Design review of the part shown in the three views and the two pictorial views. Dimensions are in mm from the part's minimum x, y and z. A direction names the side the tool comes from. Give positions to 0.01 mm unless a question says otherwise; leave off trailing zeros. Write each loop counter-clockwise with the first axis right and the second up, starting at its lowest first coordinate (ties: lowest second). Pieces come first, ordered by that corner, then holes. Notation, with made-up numbers: (-14, -37) -> (23, -37) arc R16 ccw to (23, -28) -> close; hole circle Ø10 at (67.25, 81.5). An arc over 180 degrees is marked (long way). Use CSV: the item, a comma, the result in double quotes.
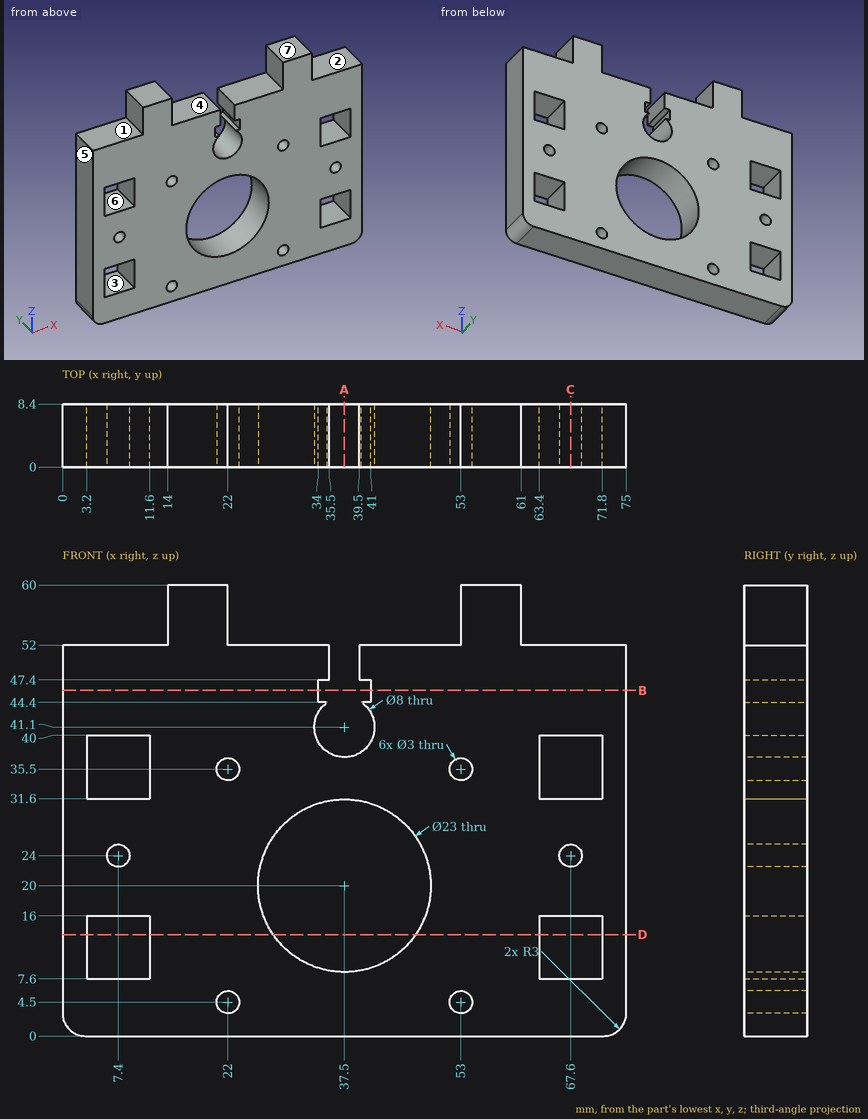
Q1. Consider section D-D (z = 13.5). Write out the cut boundary in (x, y).
Derived:
outline,"(0, 0) -> (3.2, 0) -> (3.2, 8.4) -> (0, 8.4) -> close; (11.6, 0) -> (28.01, 0) -> (28.01, 8.4) -> (11.6, 8.4) -> close; (46.99, 0) -> (63.4, 0) -> (63.4, 8.4) -> (46.99, 8.4) -> close; (71.8, 0) -> (75, 0) -> (75, 8.4) -> (71.8, 8.4) -> close"
Q2. Consider section C-C (x = 67.6). Write out the cut boundary in (y, z).
Derived:
outline,"(0, 0) -> (8.4, 0) -> (8.4, 7.6) -> (0, 7.6) -> close; (0, 16) -> (8.4, 16) -> (8.4, 22.5) -> (0, 22.5) -> close; (0, 25.5) -> (8.4, 25.5) -> (8.4, 31.6) -> (0, 31.6) -> close; (0, 40) -> (8.4, 40) -> (8.4, 52) -> (0, 52) -> close"
Q3. Consider section B-B (z = 46). Write out the cut boundary in (x, y).
Derived:
outline,"(0, 0) -> (34, 0) -> (34, 8.4) -> (0, 8.4) -> close; (41, 0) -> (75, 0) -> (75, 8.4) -> (41, 8.4) -> close"
Q4. Machinability: for the marked faces 1, 2 and 3, which of the approach directions +Z, -Z, +X, -X, +Y, -Y give a long, thin tool a straight path to every point of the face, cutting with its end or side? Answer none if there is none.
Derived:
face 1,"+Z, -X, +Y, -Y"
face 2,"+Z, +X, +Y, -Y"
face 3,"+Y, -Y"
Q5. Insertion check: pin 1 (1.5 mm diameter, centred on y = 7, z = 7, fed in from -X); pin 2 (4 mm diameter, centred on y = 5, z = 57.5, fed in from +X); pin 3 (2.5 mm diameter, centred on x = 10, y = 4, fed in from +Z); pin 4 (2.5 mm diameter, centred on x = 53, z = 4.5, fed in from -Y). Each pin has a flat end and moves straight along its axis. Give the tip position at first contact, or say it passes through.
Derived:
pin 1,"stops at x = 0"
pin 2,"stops at x = 61"
pin 3,"stops at z = 52"
pin 4,"passes through"
Q6. To check wall thickness, follow probe 1 along Z at (x, y) = (7.4, 4.5); probe 2 along X at (y, z) = (3.5, 35.5); probe 3 along X at (y, z) = (2.5, 4.5). State the ranges of each line that lie inside material, in increasing order.
Derived:
probe 1,"z = 0 to 7.6, 16 to 22.5, 25.5 to 31.6, 40 to 52"
probe 2,"x = 0 to 3.2, 11.6 to 20.5, 23.5 to 51.5, 54.5 to 63.4, 71.8 to 75"
probe 3,"x = 0 to 20.5, 23.5 to 51.5, 54.5 to 75"
Q7. The part is to be moulded in two halves that separate along X. For the marked faces 4, 5, 6 and 7, say which applies: pulls with the +X half, pulls with the -X half, needs draft (parallel to the pull), parting line crosses it, or undercut.
Derived:
face 4,"undercut"
face 5,"pulls with the -X half"
face 6,"undercut"
face 7,"needs draft"
Q8. Consider section A-A (x = 37.5). Write out the cut boundary in (y, z), then the cut area to 3 significant figures.
Derived:
outline,"(0, 0) -> (8.4, 0) -> (8.4, 8.5) -> (0, 8.5) -> close; (0, 31.5) -> (8.4, 31.5) -> (8.4, 37.1) -> (0, 37.1) -> close"
area,"118 mm2"
